Verification items for this drawing (mm, ordinates from the low corner). Coordinates: 2 decimals unless noted, no trailing zeros. Order: outer loops, then holes, each group sorted by start corner. A loop starts at its lowest first (then second) coordinate and runs counter-clockwise, first axis right, second up. Notation, with made-up numbers: (29.5, -40) -> (62.5, -40) arc R15 ccw to (62.5, -15) -> close; hole circle Ø9 at (18.25, 18.5). An arc over 180 degrees is marked (long way). Write each question's results on one line, items separated by ' | '. Start each with the question number.
(1) Draft check along X on the marked faces 1, 2, 3 and 4. Enter one of: +X half, -X half, draft (parallel to the pull), parting line (faces both ways), or undercut.
(2) Cross-section at C-C on x = 12.5. Enter the section's corners in (y, z).
(3) Thickness scan on probe 1 along X at (y, z) = (5.5, 24); probe 2 along Y at (x, z) = (15.5, 27). Record the ranges inside material, lowest first. Write a range as [from, to].
(4) Cross-section at A-A on y = 6.5. Enter the section's corners in (x, z), and give its area (4 significant figures).
(5) Cross-section at B-B on z = 3. Enter the section's corners in (x, y), and give its area (4 significant figures).
(6) Go/stop test with flat-tipped pins: pin 1 (10 mm diameter, centred on x = 13.5, z = 27, fed in from -Y); pin 2 (8 mm diameter, centred on x = 12.5, z = 13, fed in from +Y). Record where each tip stops, or that it passes through.
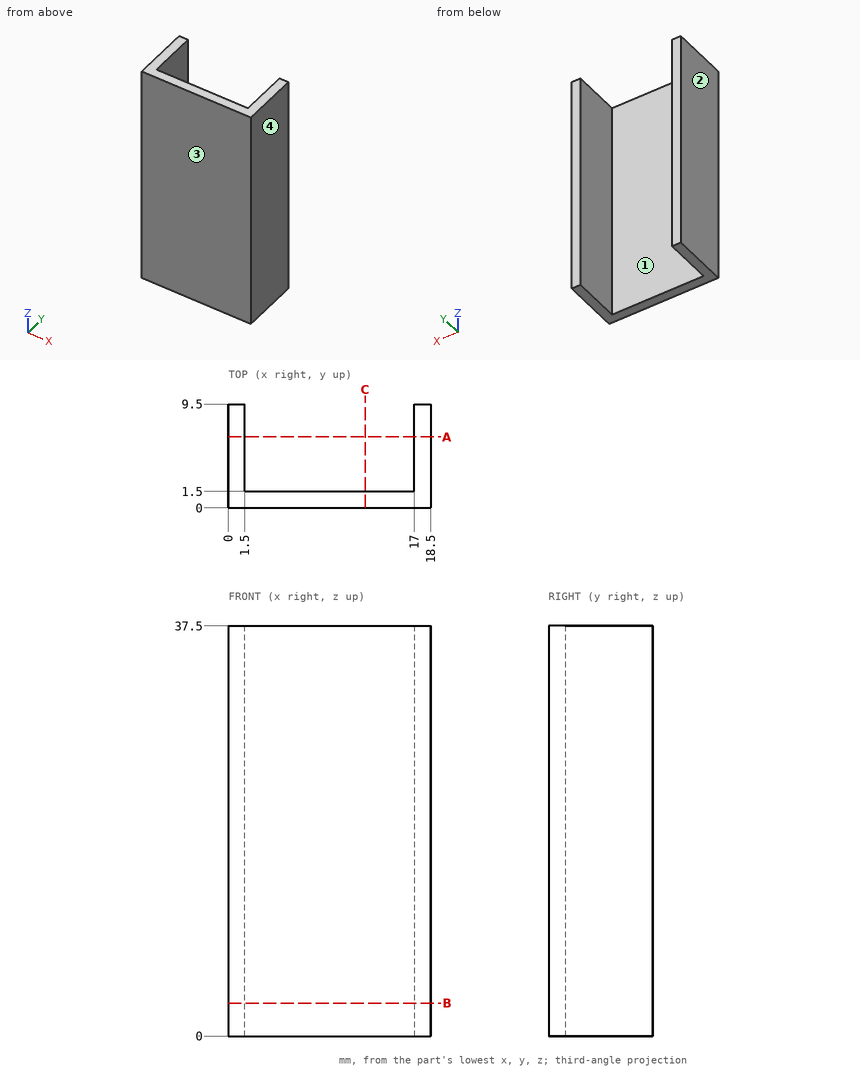
Results are:
1) face 1: undercut | face 2: -X half | face 3: draft | face 4: +X half
2) outline: (0, 0) -> (1.5, 0) -> (1.5, 37.5) -> (0, 37.5) -> close
3) probe 1: x = [0, 1.5], [17, 18.5] | probe 2: y = [0, 1.5]
4) outline: (0, 0) -> (1.5, 0) -> (1.5, 37.5) -> (0, 37.5) -> close; (17, 0) -> (18.5, 0) -> (18.5, 37.5) -> (17, 37.5) -> close | area: 112.5 mm2
5) outline: (0, 0) -> (18.5, 0) -> (18.5, 9.5) -> (17, 9.5) -> (17, 1.5) -> (1.5, 1.5) -> (1.5, 9.5) -> (0, 9.5) -> close | area: 51.75 mm2
6) pin 1: stops at y = 0 | pin 2: stops at y = 1.5
